from build123d import *

# Parameters (mm, degrees)
F0_W     = 260
F0_H     = 200
F1_DEPTH = 12
F2_DEPTH = 4
F3_W     = 15
F3_H     = 30
F4_DEPTH = 7


with BuildPart() as f1:
    # F0 (on Top) → F1 (new body)
    with BuildSketch(Plane.XY):
        Rectangle(F0_W, F0_H)
        Polygon((-98, 77.5), (98, 77.5), (118, 57.5), (118, -57.5), (98, -77.5), (30, -77.5), (-30, -77.5), (-98, -77.5), (-118, -57.5), (-118, 57.5), align=None, mode=Mode.SUBTRACT)
        with BuildLine():
            Line((118, 57.5), (98, 77.5))
            Line((98, 77.5), (-98, 77.5))
            Line((-98, 77.5), (-118, 57.5))
            Line((-118, 57.5), (-118, -57.5))
            Line((-118, -57.5), (-98, -77.5))
            Line((-98, -77.5), (-30, -77.5))
            Line((-30, -77.5), (-30, -49.638695))
            ThreePointArc((-30, -49.638695), (0, 58), (30, -49.638695))
            Line((30, -49.638695), (30, -77.5))
            Line((30, -77.5), (98, -77.5))
            Line((98, -77.5), (118, -57.5))
            Line((118, -57.5), (118, 57.5))
        make_face()
    extrude(amount=F1_DEPTH)

    # F0 (on Top) → F2 (join)
    with BuildSketch(Plane.XY):
        with BuildLine():
            Line((118, 57.5), (98, 77.5))
            Line((98, 77.5), (-98, 77.5))
            Line((-98, 77.5), (-118, 57.5))
            Line((-118, 57.5), (-118, -57.5))
            Line((-118, -57.5), (-98, -77.5))
            Line((-98, -77.5), (-30, -77.5))
            Line((-30, -77.5), (-30, -49.638695))
            ThreePointArc((-30, -49.638695), (0, 58), (30, -49.638695))
            Line((30, -49.638695), (30, -77.5))
            Line((30, -77.5), (98, -77.5))
            Line((98, -77.5), (118, -57.5))
            Line((118, -57.5), (118, 57.5))
        make_face()
    extrude(amount=-F2_DEPTH)

    # F3 (on face) → F4 (join)
    with BuildSketch(Plane.XY.offset(12)):
        with Locations((-137.5, 65)):
            Rectangle(F3_W, F3_H)
        with Locations((137.5, 65)):
            Rectangle(F3_W, F3_H)
    extrude(amount=-F4_DEPTH)


solid = f1.part
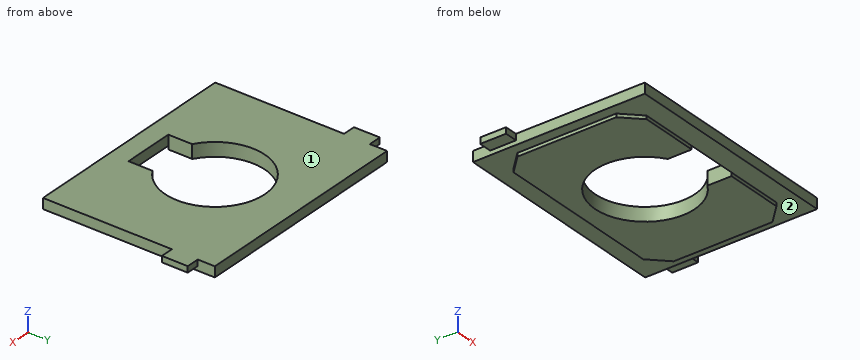
Input: part model. Units: mm. Frame: model coordinates. Face numbers are marked on the shaded views. A direction names the side the tool comes from. Round coordinates to 2 decimals unless told otherwise and drop trailing zeros. Loops run counter-clockwise (first coordinate to the right, second up) from the corner with the lowest first, then second, coordinate; pieces in that order, holes last. Notation, with made-up numbers: M -13,52.25 L 28,52.25 A22 ccw 28,90.25 Z; hole C 85.25,56.5 d3. An arc over 180 degrees is marked long. Answer as CSV lines item,"result". Start each with the question number.
(1) Line query: line 1 (X direction, y = 0, z = 8.75); line 2 (Y direction, x = 0, z = 8); line 3 (X direction, y = 65, z = 0.5). Output: solid intervals per line, ascending. Write a range as [from, to].
(2) Reachability of the marked faces 1 and 2 from +Z, -Z, +X, -X, +Y, -Y: full face, straight path, thin tool, end or side. Return the list, or none.
(3) Section B-B, the plane z = 8.25. Output: boundary loops of the cut face in (x, y).
(4) First-contact query: pin 1 (2 mm diameter, centred on y = -10, z = -2.5, fed in from -X); pin 2 (2 mm diameter, centred on y = 12.5, z = -1.5, fed in from +X); pin 3 (7.5 mm diameter, centred on x = -134, z = 8.5, fed in from -Y). Flat tips, straight axial feed; report the tip coordinate or a pass-through.
(5) Section C-C, the plane y = 0. Output: boundary loops of the cut face in (x, z), plus the area to 3 significant figures.
(6) Section A-A, the plane x = 0. Output: boundary loops of the cut face in (y, z).
(7) Section D-D, the plane x = 73.5. Output: boundary loops of the cut face in (y, z).
Values found:
1,line 1,"x = [-130, -58], [58, 130]"
1,line 2,"y = [-100, -77.5], [58, 100]"
1,line 3,"x = [-130, 130]"
2,face 1,"+Z, +X, -X, +Y, -Y"
2,face 2,"-Z"
3,outline,"M -145,50 L -130,50 L -130,-100 L 130,-100 L 130,50 L 145,50 L 145,80 L 130,80 L 130,100 L -130,100 L -130,80 L -145,80 Z; hole M -30,-77.5 L 30,-77.5 L 30,-49.64 A58 ccw long -30,-49.64 Z"
4,pin 1,"stops at x = -118"
4,pin 2,"stops at x = 118"
4,pin 3,"stops at y = 50"
5,outline,"M -130,0 L -118,0 L -118,-4 L -58,-4 L -58,12 L -130,12 Z; M 58,-4 L 118,-4 L 118,0 L 130,0 L 130,12 L 58,12 Z"
5,area,"2,210 mm²"
6,outline,"M -100,0 L -77.5,0 L -77.5,12 L -100,12 Z; M 58,-4 L 77.5,-4 L 77.5,0 L 100,0 L 100,12 L 58,12 Z"
7,outline,"M -100,0 L -77.5,0 L -77.5,-4 L 77.5,-4 L 77.5,0 L 100,0 L 100,12 L -100,12 Z"
